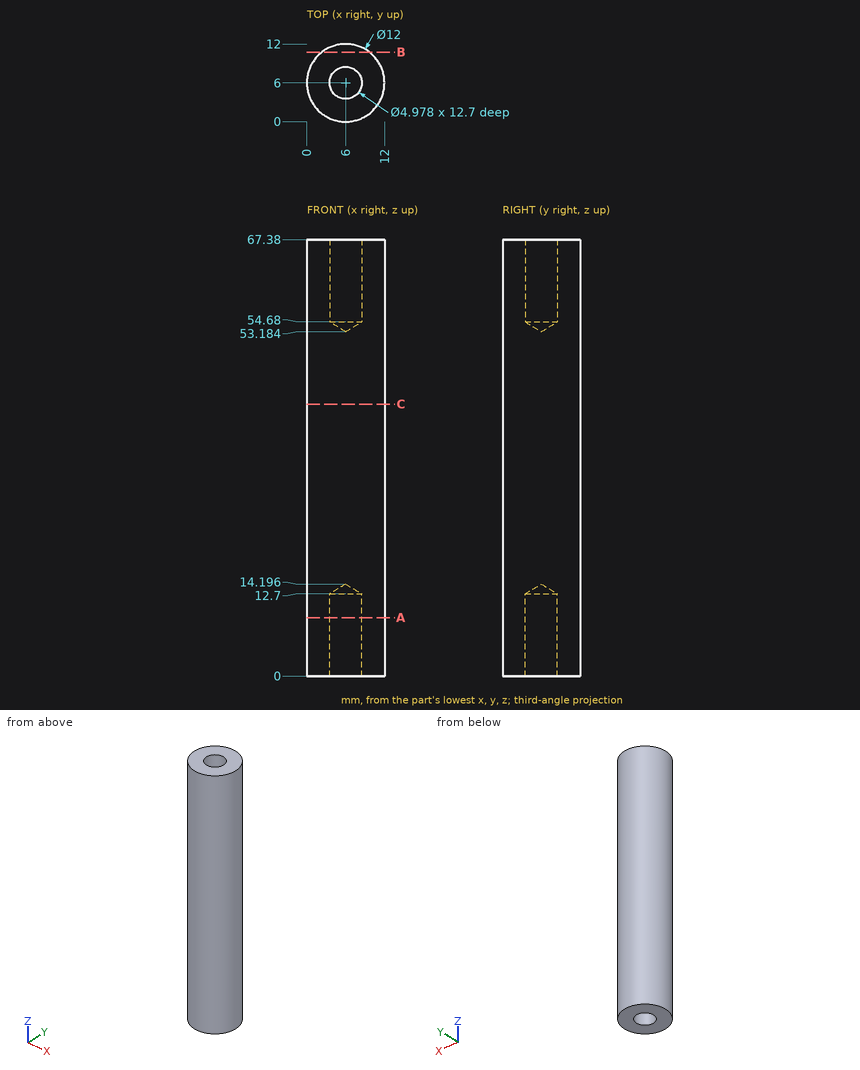
Part print with two shaded views. Sizes in mm from the minimum x, y, z corner. Round coordinates to 2 decimals unless told otherwise and drop trailing zeros. Write each loop counter-clockwise with the first axis right and the second up, starting at its lowest first coordinate (ties: lowest second). Pieces come first, ordered by that corner, then holes. Notation, with made-up numbers: M 54,8.5 L 85,8.5 A11 ccw 85,26.5 Z; hole C 29.25,-14 d1. An arc over 180 degrees is marked long. Use CSV: the item, a comma, the result in double quotes.
1. Flat gauge pins, fed straight in: pin 1 (3 mm diameter, centred on y = 8, z = 42.5, fed in from -X); pin 2 (4.5 mm diameter, centred on x = 6, y = 6, fed in from +Z). Where does each tip first touch, or does it go through?
Reply:
pin 1,"stops at x = 0.02"
pin 2,"stops at z = 54.54"
2. Wall check: probe 1 along Y at (x, z) = (6, 63.5); probe 2 along X at (y, z) = (7, 57) (1 decimal); probe 3 along Y at (x, z) = (2.75, 18) (1 decimal). Give the ranges that are in metal, low to high. Write a range as from..to.
Reply:
probe 1,"y = 0..3.51, 8.49..12"
probe 2,"x = 0.1..3.7, 8.3..11.9"
probe 3,"y = 1..11"
3. Saw through at B-B (y = 10.75). Give the cut face in (x, z) (1 decimal), plus the area to 3 significant figures.
Reply:
outline,"M 2.3,0 L 9.7,0 L 9.7,67.4 L 2.3,67.4 Z"
area,"494 mm²"
4. Saw through at A-A (z = 9). Give the cut face in (x, y).
Reply:
outline,"C 6,6 d12; hole C 6,6 d4.98"
5. Saw through at C-C (z = 42). Give the cut face in (x, y).
Reply:
outline,"C 6,6 d12"
